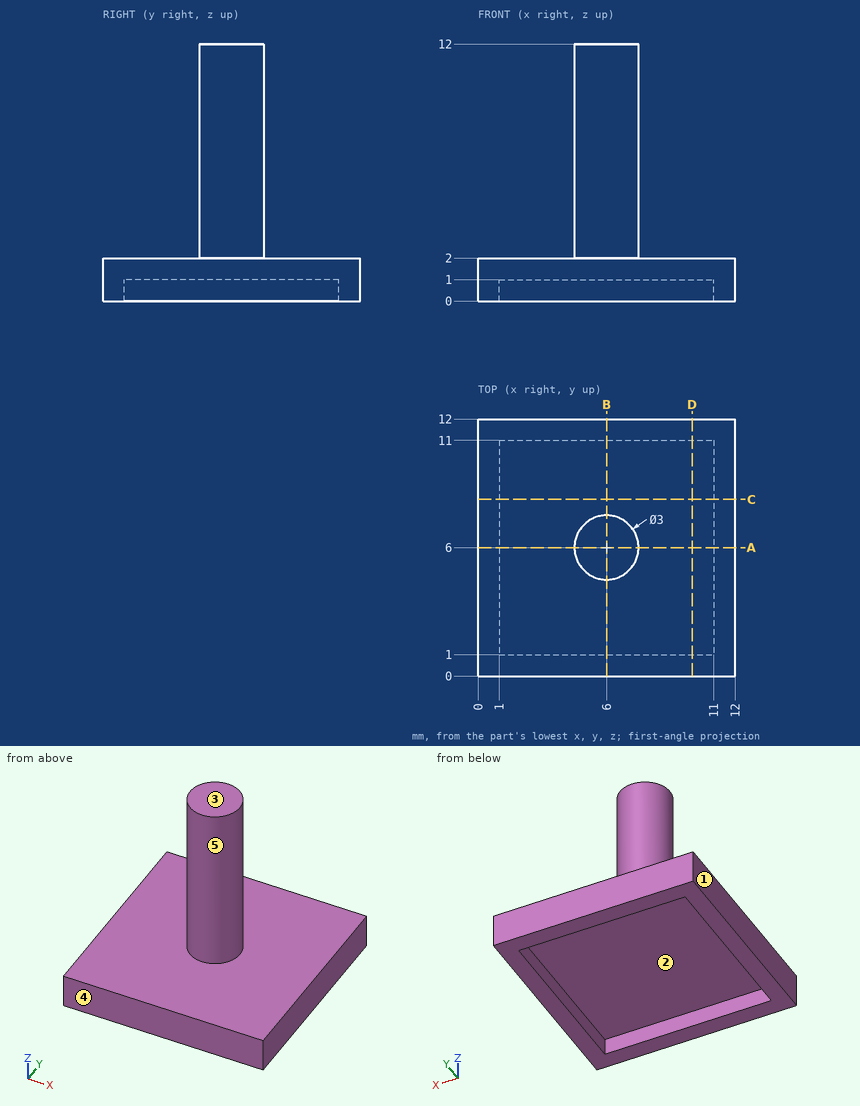
Part print with two shaded views. Sizes in mm from the minimum x, y, z corner. A direction names the side the tool comes from. Coordinates: 2 decimals unless noted, no trailing zeros. Order: outer loops, then holes, each group sorted by start corner. A loop starts at its lowest first (then second) coordinate and runs counter-clockwise, first axis right, second up. Notation, with made-up numbers: (69.25, 80) - (77.25, 80) arc R16 cw to (77.25, 103) - close; hole circle Ø5 at (54.25, 10.5). An arc over 180 degrees is marked (long way). Answer in a Markdown table with one row per item.
1. Drill centre lines: L1, parallel to Z at x = 2.75, y = 5.75; L2, parallel to Z at x = 11.75, y = 11; L3, parallel to Y at x = 6.5, z = 6.25. Where is each one in solid material? Low to high. Write a range as from..to.
Answer:
| item | result |
|---|---|
| L1 | 1..2 |
| L2 | 0..2 |
| L3 | 4.59..7.41 |
2. Slice it at A-A, the plane y = 6. List the corners of the cut face in (x, z).
Answer:
| item | result |
|---|---|
| outline | (0, 0) - (1, 0) - (1, 1) - (11, 1) - (11, 0) - (12, 0) - (12, 2) - (7.5, 2) - (7.5, 12) - (4.5, 12) - (4.5, 2) - (0, 2) - close |
3. Pull direction X, two halves, no side cores. Call the marked faces 1, 2 and 3: +X half, -X half, draft (parallel to the pull), parting line (faces both ways), or undercut.
Answer:
| item | result |
|---|---|
| face 1 | -X half |
| face 2 | undercut |
| face 3 | draft |
4. 3-axis set-ups, long thin cutter, end or side, ignore diameter. For the marked faces 4 and 5: which of +Z, -Z, +X, -X, +Y, -Y reach the whole face in a straight line?
Answer:
| item | result |
|---|---|
| face 4 | +Z, -Z, +X, -X, -Y |
| face 5 | +Z |
5. Flat gauge pins, fed straight in: P1, Ø5, axis at x = 7.5, y = 4, coming from the -Z side; P2, Ø4, axis at x = 9.5, y = 3, coming from the +Z side; P3, Ø1, axis at x = 7.5, z = 5, coming from the -Y side; P4, Ø1.1, axis at y = 5, z = 0.5, coming from the -X side. Where does each tip first touch, or does it go through?
Answer:
| item | result |
|---|---|
| P1 | z = 1 |
| P2 | z = 2 |
| P3 | y = 4.88 |
| P4 | x = 0 |
6. Slice it at C-C, the plane y = 8.25. List the corners of the cut face in (x, z).
Answer:
| item | result |
|---|---|
| outline | (0, 0) - (1, 0) - (1, 1) - (11, 1) - (11, 0) - (12, 0) - (12, 2) - (0, 2) - close |
